Verification items for the finished model (mm, model axes). Coordinates: 2 decimals unless noted, no trailing zeros. Write each loop counter-clockwise with the first axis right and the second up, starting at its lowest first coordinate (ties: lowest second). Pieces come first, ordered by that corner, then holes. Notation, with made-up numbers: (-11, 23) -> (-7, 23) arc R17 ccw to (-7, 51) -> close; hole circle Ø4 at (88, 40). An arc over 180 degrees is marked (long way). Answer in a Markdown table with one row per item.
```python
from build123d import *

# Parameters (mm, degrees)
EXTRUDE1_DEPTH          = 1.25
CUT_EXTRUDE3_DEPTH      = 2.25
LPATTERN4_COUNT         = 2
LPATTERN4_PITCH         = 2.54
SKETCH2_W               = 1.752893218
SKETCH2_H               = 0.33
CUT_EXTRUDE1_DEPTH      = 2.27
CUT_EXTRUDE1_DEPTH_BACK = 4.81
SKETCH3_W               = 11
SKETCH3_H               = 0.64
EXTRUDE_THIN1_DEPTH     = 0.32
LPATTERN5_COUNT         = 2
LPATTERN5_PITCH         = 2.54
CHAMFER2_SIZE           = 0.6
CHAMFER2_SIZE2          = 0.105796188
CHAMFER2_PART_2_SIZE    = 0.6
CHAMFER2_PART_2_SIZE2   = 0.105796188
CHAMFER2_PART_3_SIZE    = 0.6
CHAMFER2_PART_3_SIZE2   = 0.105796188
CHAMFER2_PART_4_SIZE    = 0.6
CHAMFER2_PART_4_SIZE2   = 0.105796188
CHAMFER2_PART_5_SIZE    = 0.6
CHAMFER2_PART_5_SIZE2   = 0.105796188
CHAMFER2_PART_6_SIZE    = 0.6
CHAMFER2_PART_6_SIZE2   = 0.105796188
CHAMFER2_PART_7_SIZE    = 0.6
CHAMFER2_PART_7_SIZE2   = 0.105796188
CHAMFER2_PART_8_SIZE    = 0.6
CHAMFER2_PART_8_SIZE2   = 0.105796188
CHAMFER2_PART_9_SIZE    = 0.6
CHAMFER2_PART_9_SIZE2   = 0.105796188
CHAMFER2_PART_10_SIZE   = 0.6
CHAMFER2_PART_10_SIZE2  = 0.105796188
CHAMFER2_PART_11_SIZE   = 0.6
CHAMFER2_PART_11_SIZE2  = 0.105796188
CHAMFER2_PART_12_SIZE   = 0.6
CHAMFER2_PART_12_SIZE2  = 0.105796188
CHAMFER2_PART_13_SIZE   = 0.6
CHAMFER2_PART_13_SIZE2  = 0.105796188
CHAMFER2_PART_14_SIZE   = 0.6
CHAMFER2_PART_14_SIZE2  = 0.105796188
CHAMFER2_PART_15_SIZE   = 0.6
CHAMFER2_PART_15_SIZE2  = 0.105796188
CHAMFER2_PART_16_SIZE   = 0.6
CHAMFER2_PART_16_SIZE2  = 0.105796188


with BuildPart() as part:
    # Sketch1 → Extrude1 (new body, symmetric)
    with BuildSketch(Plane.XY):
        Polygon((-1.27, 0.896446609), (-0.916446609, 1.25), (0.916446609, 1.25), (1.27, 0.896446609), (1.27, -0.896446609), (0.916446609, -1.25), (-0.916446609, -1.25), (-1.27, -0.896446609), align=None)
    extrude1 = extrude(amount=EXTRUDE1_DEPTH, both=True)

    # Sketch4 → Cut-Extrude3 (cut, symmetric)
    with BuildSketch(Plane(origin=(0, 0, 0), x_dir=(1, 0, 0), z_dir=(0, 1, 0))):
        Polygon((-1.27, -1.15), (-1.17, -1.25), (-1.27, -1.25), align=None)
        Polygon((1.17, -1.25), (1.27, -1.15), (1.27, -1.25), align=None)
    cut_extrude3 = extrude(amount=CUT_EXTRUDE3_DEPTH, both=True, mode=Mode.SUBTRACT)

    # LPattern4: Extrude1, Cut-Extrude3 ×2
    with Locations(*[(-i * LPATTERN4_PITCH, 0, 0) for i in range(1, LPATTERN4_COUNT)]):
        add(extrude1)
        add(cut_extrude3, mode=Mode.SUBTRACT)

    # Sketch2 → Cut-Extrude1 (cut, two sides)
    with BuildSketch(Plane(origin=(0, 0, 0), x_dir=(0, -1, 0), z_dir=(1, 0, 0))) as cut_extrude1_sk:
        with Locations((0, 1.085)):
            Rectangle(SKETCH2_W, SKETCH2_H)
    extrude(amount=CUT_EXTRUDE1_DEPTH, mode=Mode.SUBTRACT)
    extrude(cut_extrude1_sk.sketch, amount=-CUT_EXTRUDE1_DEPTH_BACK, mode=Mode.SUBTRACT)

    # Sketch3 → Extrude-Thin1 (add, symmetric)
    with BuildSketch(Plane(origin=(0, 0, 0), x_dir=(0, 0, -1), z_dir=(1, 0, 0))):
        with Locations((-1.75, 0)):
            Rectangle(SKETCH3_W, SKETCH3_H)
    extrude_thin1 = extrude(amount=EXTRUDE_THIN1_DEPTH, both=True)

    # LPattern5: Extrude-Thin1 ×2
    with Locations(*[(-i * LPATTERN5_PITCH, 0, 0) for i in range(1, LPATTERN5_COUNT)]):
        add(extrude_thin1)

    # Chamfer2
    chamfer2_edges = [part.edges().sort_by_distance(p)[0] for p in [
        (0, -0.32, 7.25),
    ]]
    chamfer2_side = [part.faces().sort_by_distance(p)[0] for p in [
        (0, -0.32, 4.25),
    ]]
    chamfer(chamfer2_edges, length=CHAMFER2_SIZE, length2=CHAMFER2_SIZE2, reference=chamfer2_side[0])

    # Chamfer2 part 2
    chamfer2_part_2_edges = [part.edges().sort_by_distance(p)[0] for p in [
        (0, 0.32, -3.75),
    ]]
    chamfer2_part_2_side = [part.faces().sort_by_distance(p)[0] for p in [
        (0, 0.32, -2.335),
    ]]
    chamfer(chamfer2_part_2_edges, length=CHAMFER2_PART_2_SIZE, length2=CHAMFER2_PART_2_SIZE2, reference=chamfer2_part_2_side[0])

    # Chamfer2 part 3
    chamfer2_part_3_edges = [part.edges().sort_by_distance(p)[0] for p in [
        (-0.32, 0, 7.25),
    ]]
    chamfer2_part_3_side = [part.faces().sort_by_distance(p)[0] for p in [
        (-0.32, 0, 4.25),
    ]]
    chamfer(chamfer2_part_3_edges, length=CHAMFER2_PART_3_SIZE, length2=CHAMFER2_PART_3_SIZE2, reference=chamfer2_part_3_side[0])

    # Chamfer2 part 4
    chamfer2_part_4_edges = [part.edges().sort_by_distance(p)[0] for p in [
        (-0.32, 0, -3.75),
    ]]
    chamfer2_part_4_side = [part.faces().sort_by_distance(p)[0] for p in [
        (-0.32, 0, -2.335),
    ]]
    chamfer(chamfer2_part_4_edges, length=CHAMFER2_PART_4_SIZE, length2=CHAMFER2_PART_4_SIZE2, reference=chamfer2_part_4_side[0])

    # Chamfer2 part 5
    chamfer2_part_5_edges = [part.edges().sort_by_distance(p)[0] for p in [
        (0, -0.32, -3.75),
    ]]
    chamfer2_part_5_side = [part.faces().sort_by_distance(p)[0] for p in [
        (0, -0.32, -2.335),
    ]]
    chamfer(chamfer2_part_5_edges, length=CHAMFER2_PART_5_SIZE, length2=CHAMFER2_PART_5_SIZE2, reference=chamfer2_part_5_side[0])

    # Chamfer2 part 6
    chamfer2_part_6_edges = [part.edges().sort_by_distance(p)[0] for p in [
        (0.32, 0, -3.75),
    ]]
    chamfer2_part_6_side = [part.faces().sort_by_distance(p)[0] for p in [
        (0.32, 0, -2.335),
    ]]
    chamfer(chamfer2_part_6_edges, length=CHAMFER2_PART_6_SIZE, length2=CHAMFER2_PART_6_SIZE2, reference=chamfer2_part_6_side[0])

    # Chamfer2 part 7
    chamfer2_part_7_edges = [part.edges().sort_by_distance(p)[0] for p in [
        (0, 0.32, 7.25),
    ]]
    chamfer2_part_7_side = [part.faces().sort_by_distance(p)[0] for p in [
        (0, 0.32, 4.25),
    ]]
    chamfer(chamfer2_part_7_edges, length=CHAMFER2_PART_7_SIZE, length2=CHAMFER2_PART_7_SIZE2, reference=chamfer2_part_7_side[0])

    # Chamfer2 part 8
    chamfer2_part_8_edges = [part.edges().sort_by_distance(p)[0] for p in [
        (0.32, 0, 7.25),
    ]]
    chamfer2_part_8_side = [part.faces().sort_by_distance(p)[0] for p in [
        (0.32, 0, 4.25),
    ]]
    chamfer(chamfer2_part_8_edges, length=CHAMFER2_PART_8_SIZE, length2=CHAMFER2_PART_8_SIZE2, reference=chamfer2_part_8_side[0])

    # Chamfer2 part 9
    chamfer2_part_9_edges = [part.edges().sort_by_distance(p)[0] for p in [
        (-2.54, -0.32, 7.25),
    ]]
    chamfer2_part_9_side = [part.faces().sort_by_distance(p)[0] for p in [
        (-2.54, -0.32, 4.25),
    ]]
    chamfer(chamfer2_part_9_edges, length=CHAMFER2_PART_9_SIZE, length2=CHAMFER2_PART_9_SIZE2, reference=chamfer2_part_9_side[0])

    # Chamfer2 part 10
    chamfer2_part_10_edges = [part.edges().sort_by_distance(p)[0] for p in [
        (-2.54, 0.32, -3.75),
    ]]
    chamfer2_part_10_side = [part.faces().sort_by_distance(p)[0] for p in [
        (-2.54, 0.32, -2.335),
    ]]
    chamfer(chamfer2_part_10_edges, length=CHAMFER2_PART_10_SIZE, length2=CHAMFER2_PART_10_SIZE2, reference=chamfer2_part_10_side[0])

    # Chamfer2 part 11
    chamfer2_part_11_edges = [part.edges().sort_by_distance(p)[0] for p in [
        (-2.86, 0, -3.75),
    ]]
    chamfer2_part_11_side = [part.faces().sort_by_distance(p)[0] for p in [
        (-2.86, 0, -2.335),
    ]]
    chamfer(chamfer2_part_11_edges, length=CHAMFER2_PART_11_SIZE, length2=CHAMFER2_PART_11_SIZE2, reference=chamfer2_part_11_side[0])

    # Chamfer2 part 12
    chamfer2_part_12_edges = [part.edges().sort_by_distance(p)[0] for p in [
        (-2.86, 0, 7.25),
    ]]
    chamfer2_part_12_side = [part.faces().sort_by_distance(p)[0] for p in [
        (-2.86, 0, 4.25),
    ]]
    chamfer(chamfer2_part_12_edges, length=CHAMFER2_PART_12_SIZE, length2=CHAMFER2_PART_12_SIZE2, reference=chamfer2_part_12_side[0])

    # Chamfer2 part 13
    chamfer2_part_13_edges = [part.edges().sort_by_distance(p)[0] for p in [
        (-2.54, -0.32, -3.75),
    ]]
    chamfer2_part_13_side = [part.faces().sort_by_distance(p)[0] for p in [
        (-2.54, -0.32, -2.335),
    ]]
    chamfer(chamfer2_part_13_edges, length=CHAMFER2_PART_13_SIZE, length2=CHAMFER2_PART_13_SIZE2, reference=chamfer2_part_13_side[0])

    # Chamfer2 part 14
    chamfer2_part_14_edges = [part.edges().sort_by_distance(p)[0] for p in [
        (-2.22, 0, -3.75),
    ]]
    chamfer2_part_14_side = [part.faces().sort_by_distance(p)[0] for p in [
        (-2.22, 0, -2.335),
    ]]
    chamfer(chamfer2_part_14_edges, length=CHAMFER2_PART_14_SIZE, length2=CHAMFER2_PART_14_SIZE2, reference=chamfer2_part_14_side[0])

    # Chamfer2 part 15
    chamfer2_part_15_edges = [part.edges().sort_by_distance(p)[0] for p in [
        (-2.54, 0.32, 7.25),
    ]]
    chamfer2_part_15_side = [part.faces().sort_by_distance(p)[0] for p in [
        (-2.54, 0.32, 4.25),
    ]]
    chamfer(chamfer2_part_15_edges, length=CHAMFER2_PART_15_SIZE, length2=CHAMFER2_PART_15_SIZE2, reference=chamfer2_part_15_side[0])

    # Chamfer2 part 16
    chamfer2_part_16_edges = [part.edges().sort_by_distance(p)[0] for p in [
        (-2.22, 0, 7.25),
    ]]
    chamfer2_part_16_side = [part.faces().sort_by_distance(p)[0] for p in [
        (-2.22, 0, 4.25),
    ]]
    chamfer(chamfer2_part_16_edges, length=CHAMFER2_PART_16_SIZE, length2=CHAMFER2_PART_16_SIZE2, reference=chamfer2_part_16_side[0])


solid = part.part
```
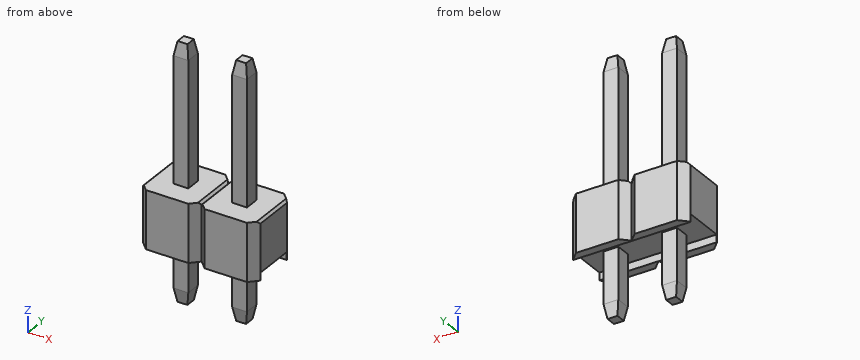
1. Sectioned sample at B-B, the plane y = -0.45. Record the cut outline in (x, z), and give its area (3 significant figures).
Findings below:
| item | result |
|---|---|
| outline | (-3.81, -0.92) -> (1.27, -0.92) -> (1.27, 1.15) -> (1.17, 1.25) -> (-1.17, 1.25) -> (-1.27, 1.15) -> (-1.37, 1.25) -> (-3.71, 1.25) -> (-3.81, 1.15) -> close |
| area | 11.0 mm² |
2. Sectioned sample at C-C, the plane y = 1.1. Record the cut outline in (x, z).
Findings below:
| item | result |
|---|---|
| outline | (-3.61, -1.25) -> (-1.47, -1.25) -> (-1.47, 1.25) -> (-3.61, 1.25) -> close; (-1.07, -1.25) -> (1.07, -1.25) -> (1.07, 1.25) -> (-1.07, 1.25) -> close |
3. Sectioned sample at D-D, the plane z = -0.75. Record the cut outline in (x, y).
Findings below:
| item | result |
|---|---|
| outline | (-3.81, -0.9) -> (-3.46, -1.25) -> (-1.62, -1.25) -> (-1.27, -0.9) -> (-0.92, -1.25) -> (0.92, -1.25) -> (1.27, -0.9) -> (1.27, 0.9) -> (0.92, 1.25) -> (-0.92, 1.25) -> (-1.27, 0.9) -> (-1.62, 1.25) -> (-3.46, 1.25) -> (-3.81, 0.9) -> close |
4. Sectioned sample at A-A, the plane z = 6.5. Record the cut outline in (x, y), and give its area (3 significant figures).
Findings below:
| item | result |
|---|---|
| outline | (-2.86, -0.32) -> (-2.22, -0.32) -> (-2.22, 0.32) -> (-2.86, 0.32) -> close; (-0.32, -0.32) -> (0.32, -0.32) -> (0.32, 0.32) -> (-0.32, 0.32) -> close |
| area | 0.819 mm² |
5. Material ranges on probe 1 along X at (y, z) = (0.15, 5.5); probe 2 along Z at (x, y) = (0.5, -0.1); probe 3 along Y at (x, z) = (-2.65, -3), recorded low to high. Write a range as from..to.
Findings below:
| item | result |
|---|---|
| probe 1 | x = -2.86..-2.22, -0.32..0.32 |
| probe 2 | z = -0.92..1.25 |
| probe 3 | y = -0.32..0.32 |
6. Go/stop test with flat-tipped pins: pin 1 (0.7 mm diameter, centred on x = 0, z = -2.5, fed in from +Y); pin 2 (0.5 mm diameter, centred on y = 0, z = 3, fed in from -X); pin 3 (1 mm diameter, centred on x = 0.5, z = 3.5, fed in from -Y). Record where each tip stops, or that it passes through.
Findings below:
| item | result |
|---|---|
| pin 1 | stops at y = 0.32 |
| pin 2 | stops at x = -2.86 |
| pin 3 | stops at y = -0.32 |
